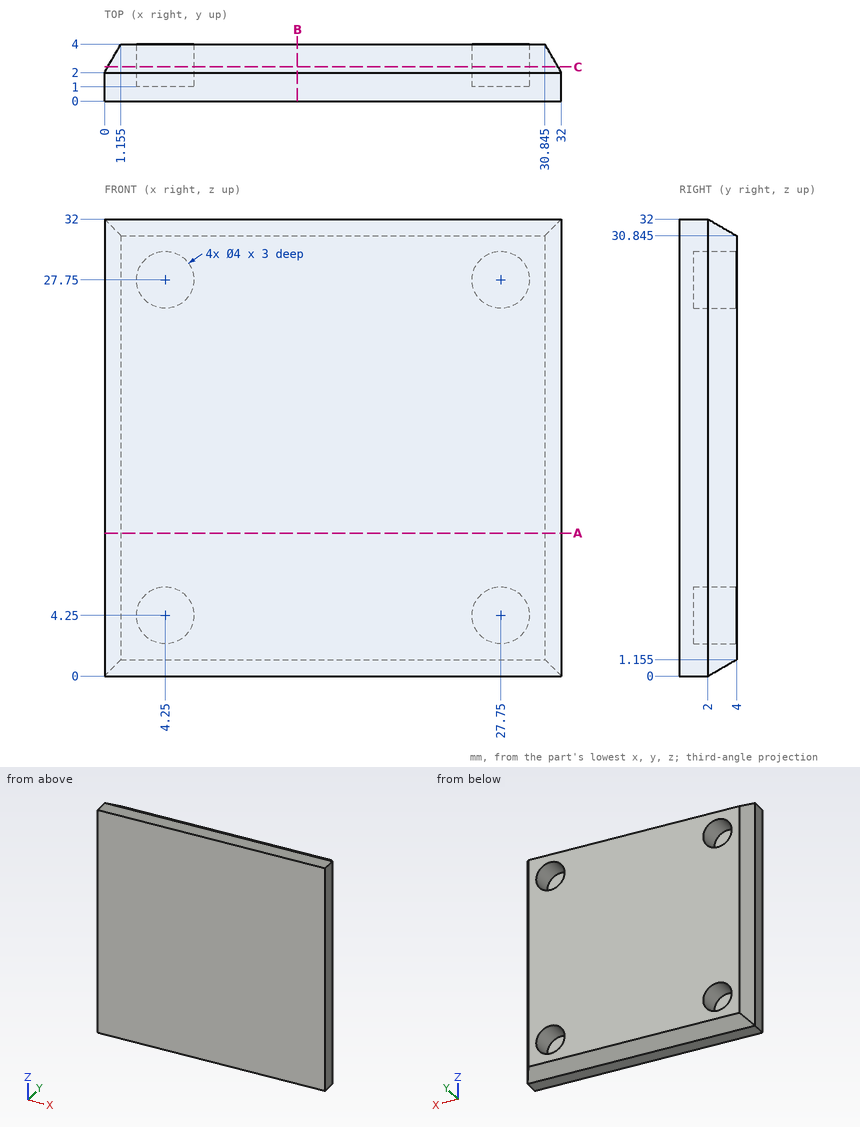
Here's the drawing with two shaded views (mm, measured from the low corner). I have some questions. Give positions to 0.01 mm unless a question says otherwise; leave off trailing zeros. Write each loop counter-clockwise with the first axis right and the second up, starting at its lowest first coordinate (ties: lowest second). Pieces come first, ordered by that corner, then holes. Notation, with made-up numbers: (74.25, 9.25) -> (112.25, 9.25) arc R20 cw to (112.25, 19.25) -> close; hole circle Ø9 at (18.5, 54.25). An arc over 180 degrees is marked (long way). Answer as a JSON object with one key per item and string values. Group by question number.
Item 1: Suppose I cut it at B-B (x = 13.5). Please give me the cut outline in (y, z) (1 decimal), plus the area to 3 significant figures.
Item 2: Please list where these lines run through material, in increasing order: line 1 (Z direction, x = 27.75, y = 2.6); line 2 (Z direction, x = 27.75, y = 3.35); line 3 (X direction, y = 2.95, z = 28) (1 decimal). Write a range as [from, to].
Item 3: I'm going to push a flat-ended pin straight in: P1, Ø2, axis at x = 4.5, z = 3.5, coming from the +Y side. Where does the tip first touch, or does it pass through?
Item 4: Suppose I cut it at A-A (z = 10). Please give me the cut outline in (x, y) (1 decimal).
Item 5: Suppose I cut it at C-C (y = 2.4). Please give me the cut outline in (x, z).
Findings:
{
 "1": {"outline": "(0, 0) -> (2, 0) -> (4, 1.2) -> (4, 30.8) -> (2, 32) -> (0, 32) -> close", "area": "126 mm²"},
 "2": {"line 1": "z = [0.35, 2.25], [6.25, 25.75], [29.75, 31.65]", "line 2": "z = [0.78, 2.25], [6.25, 25.75], [29.75, 31.22]", "line 3": "x = [0.5, 2.3], [6.2, 25.8], [29.7, 31.5]"},
 "3": {"P1": "stops at y = 1"},
 "4": {"outline": "(0, 0) -> (32, 0) -> (32, 2) -> (30.8, 4) -> (1.2, 4) -> (0, 2) -> close"},
 "5": {"outline": "(0.23, 0.23) -> (31.77, 0.23) -> (31.77, 31.77) -> (0.23, 31.77) -> close; hole circle Ø4 at (4.25, 4.25); hole circle Ø4 at (4.25, 27.75); hole circle Ø4 at (27.75, 4.25); hole circle Ø4 at (27.75, 27.75)"}
}
